Part model, mm, in its own coordinate system. A direction names the side the tool comes from. Coordinates: 2 decimals unless noted, no trailing zeros. Write each loop counter-clockwise with the first axis right and the second up, starting at its lowest first coordinate (ties: lowest second). Pieces come first, ordered by that corner, then holes. Notation, with made-up numbers: (-16.5, 18) - (38.5, 18) arc R25 cw to (38.5, 31) - close; hole circle Ø8 at (77, 86.25). An arc over 180 degrees is marked (long way). Write each question's results on one line, items separated by ' | '.
from build123d import *

# Parameters (mm, degrees)
SKETCH1_R           = 1.25
SKETCH1_W           = 8
SKETCH1_H           = 6
BOSS_EXTRUDE1_DEPTH = 9
FILLET1_R           = 7.5
FILLET2_R           = 1
BOSS_EXTRUDE2_DEPTH = 12.7
SKETCH3_W           = 2
SKETCH3_H           = 4
SKETCH3_H_2         = 3.1
SKETCH5_R           = 1.75
CUT_EXTRUDE1_DEPTH  = 10
SKETCH6_R           = 2.35
CUT_EXTRUDE2_DEPTH  = 5
SKETCH7_W           = 2.5
SKETCH7_H           = 4
CUT_EXTRUDE3_DEPTH  = 1.25
FILLET3_R           = 1.25
FILLET4_R           = 1
SKETCH8_W           = 11
SKETCH8_H           = 2.5
CUT_EXTRUDE4_DEPTH  = 1.25
FILLET5_R           = 1.25
FILLET6_R           = 1
SKETCH9_R           = 1.5
CUT_EXTRUDE5_DEPTH  = 8
SKETCH9_3_R         = 2.35
CUT_EXTRUDE6_DEPTH  = 5
SKETCH9_4_R         = 1.25
CUT_EXTRUDE7_DEPTH  = 23
SKETCH10_R          = 1.5
CUT_EXTRUDE8_DEPTH  = 8
SKETCH11_W          = 11
SKETCH11_H          = 35
CUT_EXTRUDE9_DEPTH  = 3.5
SKETCH13_W          = 9.4
SKETCH13_H          = 12
CUT_EXTRUDE10_DEPTH = 1.5
CUT_EXTRUDE11_DEPTH = 33
SKETCH15_W          = 2
SKETCH15_H          = 6
CUT_EXTRUDE12_DEPTH = 1.5
FILLET7_R           = 1
SKETCH16_W          = 8
SKETCH16_H          = 6
CUT_EXTRUDE13_DEPTH = 7.5
CUT_EXTRUDE14_DEPTH = 6
FILLET8_R           = 1


with BuildPart() as part:
    # Sketch1 → Boss-Extrude1 (new body)
    with BuildSketch(Plane.XY):
        Polygon((-27.5, 17.25), (-13, 17.25), (-13, 47.75), (2, 47.75), (2, 17.25), (27.5, 17.25), (27.5, -47.75), (-27.5, -47.75), align=None)
        with Locations((-5.5, 40.85)):
            Circle(SKETCH1_R, mode=Mode.SUBTRACT)
        with Locations((-22, -24.75)):
            Circle(SKETCH1_R, mode=Mode.SUBTRACT)
        with Locations((-15, -42.75)):
            Circle(SKETCH1_R, mode=Mode.SUBTRACT)
        with Locations(Location((15, -42.75, 0), (0, 0, 180))):
            Circle(SKETCH1_R, mode=Mode.SUBTRACT)
        with Locations(Location((22, -24.75, 0), (0, 0, 180))):
            Circle(SKETCH1_R, mode=Mode.SUBTRACT)
        with BuildLine():
            Line((-3, 33.35), (-3, 20.85))
            ThreePointArc((-3, 20.85), (-5.5, 18.35), (-8, 20.85))
            Line((-8, 20.85), (-8, 33.35))
            ThreePointArc((-8, 33.35), (-5.5, 35.85), (-3, 33.35))
        make_face(mode=Mode.SUBTRACT)
        with Locations((22, -33.75)):
            Rectangle(SKETCH1_W, SKETCH1_H, mode=Mode.SUBTRACT)
    extrude(amount=BOSS_EXTRUDE1_DEPTH)

    # Fillet1
    fillet1_edges = [part.edges().sort_by_distance(p)[0] for p in [
        (-13, 47.75, 4.5),
        (2, 47.75, 4.5),
    ]]
    fillet(fillet1_edges, radius=FILLET1_R - 0.0001)  # a hair under: the kernel refuses the full size

    # Fillet2
    fillet2_edges = [part.edges().sort_by_distance(p)[0] for p in [
        (-27.5, 17.25, 4.5),
        (-13, 17.25, 4.5),
        (2, 17.25, 4.5),
        (27.5, 17.25, 4.5),
        (27.5, -47.75, 4.5),
        (-27.5, -47.75, 4.5),
    ]]
    fillet(fillet2_edges, radius=FILLET2_R)

    # Sketch2 → Boss-Extrude2 (add)
    with BuildSketch(Plane(origin=(0, -14.35, 0), x_dir=(-1, 0, 0), z_dir=(0, -1, 0))):
        with BuildLine():
            Line((27.5, -9), (10, -9))
            Line((10, -9), (10, -24.2))
            Line((10, -24.2), (-10, -24.2))
            Line((-10, -24.2), (-10, -9))
            Line((-10, -9), (-27.5, -9))
            Line((-27.5, -9), (-27.5, -31))
            Line((-27.5, -31), (-26.263139721, -31))
            ThreePointArc((-26.263139721, -31), (-18.495572929, -29.143111899), (-17.062940163, -37))
            Line((-17.062940163, -37), (-6.25, -37))
            Line((-6.25, -37), (-6.25, -33.75))
            ThreePointArc((-6.25, -33.75), (0, -27.5), (6.25, -33.75))
            Line((6.25, -33.75), (6.25, -37))
            Line((6.25, -37), (27.5, -37))
            Line((27.5, -37), (27.5, -9))
        make_face()
    extrude(amount=-BOSS_EXTRUDE2_DEPTH)

    # Cut-Sweep1: sweep along a path in Sketch4
    with BuildLine(Plane(origin=(0, -1.65, 0), x_dir=(1, 0, 0), z_dir=(0, 1, 0))) as cut_sweep1_path:
        Line((-6.25, -37), (-6.25, -33.75))
        ThreePointArc((-6.25, -33.75), (0, -27.5), (6.25, -33.75))
        Line((6.25, -33.75), (6.25, -37))
    # Sketch3 → Cut-Sweep1 (sweep, cut)
    with BuildSketch(Plane.XY.offset(37)):
        with Locations((-7.25, -3.65)):
            Rectangle(SKETCH3_W, SKETCH3_H)
        with Locations((-7.25, -12.8)):
            Rectangle(SKETCH3_W, SKETCH3_H_2)
    sweep(path=cut_sweep1_path.line, mode=Mode.SUBTRACT)

    # Sketch5 → Cut-Extrude1 (cut)
    with BuildSketch(Plane.XY.offset(37)):
        with Locations((-12.5, -8)):
            Circle(SKETCH5_R)
        with Locations(Location((12.5, -8, 0), (0, 0, 180))):
            Circle(SKETCH5_R)
    extrude(amount=-CUT_EXTRUDE1_DEPTH, mode=Mode.SUBTRACT)

    # Sketch6 → Cut-Extrude2 (cut)
    with BuildSketch(Plane.XY.offset(37)):
        with Locations((-12.5, -8)):
            Circle(SKETCH6_R)
        with Locations((12.5, -8)):
            Circle(SKETCH6_R)
    extrude(amount=-CUT_EXTRUDE2_DEPTH, mode=Mode.SUBTRACT)

    # Sketch7 → Cut-Extrude3 (cut)
    with BuildSketch(Plane(origin=(-10, 0, 0), x_dir=(0, 0, -1), z_dir=(1, 0, 0))):
        with Locations((-16.6, -3.65)):
            Rectangle(SKETCH7_W, SKETCH7_H)
    extrude(amount=-CUT_EXTRUDE3_DEPTH, mode=Mode.SUBTRACT)

    # Fillet3
    fillet3_edges = [part.edges().sort_by_distance(p)[0] for p in [
        (-11.25, -3.65, 17.85),
        (-11.25, -3.65, 15.35),
    ]]
    fillet(fillet3_edges, radius=FILLET3_R - 0.0001)  # a hair under: the kernel refuses the full size

    # Fillet4
    fillet4_edges = [part.edges().sort_by_distance(p)[0] for p in [
        (-10.883912766, -5.65, 15.716087234),
        (-10.883912766, -5.65, 17.483912766),
    ]]
    fillet(fillet4_edges, radius=FILLET4_R)

    # Sketch8 → Cut-Extrude4 (cut)
    with BuildSketch(Plane(origin=(0, -1.65, 0), x_dir=(1, 0, 0), z_dir=(0, 1, 0))):
        with Locations((18.5, -15.6)):
            Rectangle(SKETCH8_W, SKETCH8_H)
    extrude(amount=-CUT_EXTRUDE4_DEPTH, mode=Mode.SUBTRACT)

    # Fillet5
    fillet5_edges = [part.edges().sort_by_distance(p)[0] for p in [
        (18.5, -2.9, 16.85),
        (18.5, -2.9, 14.35),
    ]]
    fillet(fillet5_edges, radius=FILLET5_R - 0.0001)  # a hair under: the kernel refuses the full size

    # Fillet6
    fillet6_edges = [part.edges().sort_by_distance(p)[0] for p in [
        (24, -2.533912766, 14.716087234),
        (24, -2.533912766, 16.483912766),
        (13, -2.533912766, 14.716087234),
        (13, -2.533912766, 16.483912766),
    ]]
    fillet(fillet6_edges, radius=FILLET6_R)

    # Sketch9 → Cut-Extrude5 (cut)
    with BuildSketch(Plane(origin=(0, 0, 0), x_dir=(-1, 0, 0), z_dir=(0, 0, -1))):
        with Locations((-12, -3.25)):
            Circle(SKETCH9_R)
        with Locations((-12, -27.25)):
            Circle(SKETCH9_R)
        with Locations(Location((12, -27.25, 0), (0, 0, 180))):
            Circle(SKETCH9_R)
        with Locations(Location((12, -3.25, 0), (0, 0, 180))):
            Circle(SKETCH9_R)
    extrude(amount=-CUT_EXTRUDE5_DEPTH, mode=Mode.SUBTRACT)

    # Sketch9<3> → Cut-Extrude6 (cut)
    with BuildSketch(Plane(origin=(0, 0, 0), x_dir=(-1, 0, 0), z_dir=(0, 0, -1))):
        with Locations((0, -15.25)):
            Circle(SKETCH9_3_R)
    extrude(amount=-CUT_EXTRUDE6_DEPTH, mode=Mode.SUBTRACT)

    # Sketch9<4> → Cut-Extrude7 (cut)
    with BuildSketch(Plane(origin=(0, 0, 0), x_dir=(-1, 0, 0), z_dir=(0, 0, -1))):
        with Locations((-22, -5.75)):
            Circle(SKETCH9_4_R)
        with Locations(Location((22, -5.75, 0), (0, 0, 180))):
            Circle(SKETCH9_4_R)
    extrude(amount=-CUT_EXTRUDE7_DEPTH, mode=Mode.SUBTRACT)

    # Sketch10 → Cut-Extrude8 (cut)
    with BuildSketch(Plane(origin=(0, 0, 0), x_dir=(-1, 0, 0), z_dir=(0, 0, -1))):
        with Locations((0, -15.25)):
            Circle(SKETCH10_R)
    extrude(amount=-CUT_EXTRUDE8_DEPTH, mode=Mode.SUBTRACT)

    # Sketch11 → Cut-Extrude9 (cut)
    with BuildSketch(Plane(origin=(0, 0, 0), x_dir=(-1, 0, 0), z_dir=(0, 0, -1))):
        with Locations((-22, -19.25)):
            Rectangle(SKETCH11_W, SKETCH11_H)
    cut_extrude9 = extrude(amount=-CUT_EXTRUDE9_DEPTH, mode=Mode.SUBTRACT)

    # Sketch13 → Cut-Extrude10 (cut)
    with BuildSketch(Plane(origin=(0, 0, 3.5), x_dir=(-1, 0, 0), z_dir=(0, 0, -1))):
        with Locations((-22, -15.25)):
            Rectangle(SKETCH13_W, SKETCH13_H)
    cut_extrude10 = extrude(amount=-CUT_EXTRUDE10_DEPTH, mode=Mode.SUBTRACT)

    # Mirror1: Cut-Extrude9, Cut-Extrude10 across plane
    add(cut_extrude9.mirror(Plane(origin=(0, 0, 0), x_dir=(0, 0, 1), z_dir=(1, 0, 0))), mode=Mode.SUBTRACT)
    add(cut_extrude10.mirror(Plane(origin=(0, 0, 0), x_dir=(0, 0, 1), z_dir=(1, 0, 0))), mode=Mode.SUBTRACT)

    # Sketch12 → Cut-Extrude11 (cut)
    with BuildSketch(Plane(origin=(16.5, 0, 0), x_dir=(0, 0, -1), z_dir=(1, 0, 0))):
        Polygon((-3.5, -30.75), (-2.5, -30.75), (-2.5, -36.75), (-5.5, -36.75), (-5.5, -30.75), align=None)
    extrude(amount=-CUT_EXTRUDE11_DEPTH, mode=Mode.SUBTRACT)

    # Sketch15 → Cut-Extrude12 (cut)
    with BuildSketch(Plane(origin=(18, 0, 0), x_dir=(0, 0, -1), z_dir=(1, 0, 0))):
        with Locations((-4.5, -33.75)):
            Rectangle(SKETCH15_W, SKETCH15_H)
    extrude(amount=-CUT_EXTRUDE12_DEPTH, mode=Mode.SUBTRACT)

    # Fillet7
    fillet7_edges = [part.edges().sort_by_distance(p)[0] for p in [
        (27.5, -36.75, 1.75),
        (27.5, -1.75, 1.75),
        (18, -30.75, 7.25),
        (-27.5, -1.75, 1.75),
        (-27.5, -36.75, 1.75),
        (18, -36.75, 7.25),
        (26, -36.75, 6.25),
        (26, -30.75, 6.25),
    ]]
    fillet(fillet7_edges, radius=FILLET7_R)

    # Sketch16 → Cut-Extrude13 (cut)
    with BuildSketch(Plane(origin=(0, 0, 0), x_dir=(-1, 0, 0), z_dir=(0, 0, -1))):
        with Locations((22, -33.75)):
            Rectangle(SKETCH16_W, SKETCH16_H)
    extrude(amount=-CUT_EXTRUDE13_DEPTH, mode=Mode.SUBTRACT)

    # Sketch17 → Cut-Extrude14 (cut)
    with BuildSketch(Plane(origin=(0, -36.75, 0), x_dir=(1, 0, 0), z_dir=(0, 1, 0))):
        Polygon((-18, -7.5), (-18, -3.5), (-16.5, -3.5), (-16.5, -5.5), align=None)
    extrude(amount=CUT_EXTRUDE14_DEPTH, mode=Mode.SUBTRACT)

    # Fillet8
    fillet8_edges = [part.edges().sort_by_distance(p)[0] for p in [
        (-27.5, -1.65, 23),
        (27.5, -1.65, 20),
        (-27.5, -14.35, 23),
        (27.5, -14.35, 20),
    ]]
    fillet(fillet8_edges, radius=FILLET8_R)


solid = part.part
(1) Saw through at B-B on x = -22. Write the cut outline in (y, z), then the cut area to 3 significant figures.
Return value:
outline: (-47.75, 0) - (-36.75, 0) - (-36.75, 7.5) - (-30.75, 7.5) - (-30.75, 3.5) - (-26, 3.5) - (-26, 9) - (-47.75, 9) - close; (-23.5, 3.5) - (-21.25, 3.5) - (-21.25, 5) - (-9.25, 5) - (-9.25, 3.5) - (-7, 3.5) - (-7, 23) - (-4.5, 23) - (-4.5, 3.5) - (-1.75, 3.5) - (-1.75, 0) - (17.25, 0) - (17.25, 9) - (-1.65, 9) - (-1.65, 37) - (-14.35, 37) - (-14.35, 9) - (-23.5, 9) - close | area: 714 mm^2
(2) Saw through at A-A on z = 20.5. Write the cut outline in (x, y), then the cut area to 3 significant figures.
Return value:
outline: (-27.5, -13.35) arc R1 ccw to (-26.5, -14.35) - (-10, -14.35) - (-10, -1.65) - (-26.5, -1.65) arc R1 ccw to (-27.5, -2.65) - close; (10, -14.35) - (26.5, -14.35) arc R1 ccw to (27.5, -13.35) - (27.5, -2.65) arc R1 ccw to (26.5, -1.65) - (10, -1.65) - close; hole circle Ø2.5 at (-22, -5.75); hole circle Ø2.5 at (22, -5.75) | area: 434 mm^2
(3) Wall check: line 1 (X direction, y = -5.5, z = 8.5); line 2 (X direction, y = -13, z = 12); line 3 (Z direction, x = 7, y = -31). Give the ranges that are in metal, low to high. Write a range as from..to.
Return value:
line 1: x = -27.5..-23.22, -20.78..20.78, 23.22..27.5 | line 2: x = -27.5..-10, 10..27.5 | line 3: z = 0..2.5, 5.5..9
(4) Two-plate mould, pull along Y, no slides. Class faces 5 (the flat face through (0, -5.65, 27)), 6 (the flat face through (-8.25, -4, 35)), 7 (the flat face through (13, -8, 27)): released by +Y, released by -Y, zero draft, split by the parting line, or undercut.
Return value:
face 5: released by +Y | face 6: zero draft | face 7: undercut
(5) Flat gauge pins, fed straight in: P1, Ø1.6, axis at y = -3.5, z = 35.5, coming from the +X side; P2, Ø3.5, axis at y = -8.5, z = 36, coming from the +X side; P3, Ø4, axis at x = 22, y = -24.75, coming from the +Z side. Where does each tip first touch, or does it go through?
Return value:
P1: stops at x = 16.63 | P2: stops at x = 17.06 | P3: stops at z = 9
(6) 3-axis set-ups, long thin cutter, end or side, ignore diameter. For faces 1 (the flat face through (22, -1.75, 2)), 2 (the flat face through (-13, -6, 32)), 3 (the flat face through (10, -8, 17)), 4 (the cylindrical face through (-21, -5, 13)): which of +Z, -Z, +X, -X, +Y, -Y reach the whole face in a straight line?
Return value:
face 1: -Z, +X | face 2: +Z | face 3: +Y, -Y | face 4: -Z
(7) Saw through at C-C on y = 32. Write the cut outline in (x, z), then the cut area to 3 significant figures.
Return value:
outline: (-13, 0) - (-8, 0) - (-8, 9) - (-13, 9) - close; (-3, 0) - (2, 0) - (2, 9) - (-3, 9) - close | area: 90.0 mm^2
